Here's how the part is built. I have some questions about the finished solid (model axes, mm). A direction names the side the tool comes from. Coordinates: 2 decimals unless noted, no trailing zeros. Loops run counter-clockwise (first coordinate to the right, second up) from the corner with the lowest first, then second, coordinate; pieces in that order, holes last. Notation, with made-up numbers: M -11,66.25 L 9,66.25 A19 ccw 9,87.25 Z; hole C 77.5,66.5 d10. An arc over 180 degrees is marked long. Use CSV: the item, a comma, the result in double quotes. Start each with the question number.
Q1. Please list where these lines run through material, in increasing order: probe 1 along X at (y, z) = (3.5, 25); probe 2 along Z at (x, y) = (77.5, 6.25); probe 3 along X at (y, z) = (3.5, -15). Write a range as [from, to].
Q2. If we section it at A-A (x = 90): Please give me the cut outline in (y, z), and give its area (3 significant figures).
Q3. For pin 1 Ø2 at (x, z) = (100, 25) entering from +Y; pin 2 Ø4.5 at (x, z) = (-77.5, 14.5) entering from +Y, each with a flat end and sliding along its axis, tell me the tip position at first contact or that it passes through.
Q4. If we mould it in two halves opening along X, with no side actions, what happens to faces 6 (the flat face through (23, 10, -13)), 7 (the cylindrical face through (100.354, 3.402, -13.176))? For each: +X half, -X half, draft (parallel to the pull), parting line (faces both ways), or undercut.
Q5. Which directions (+Z, -Z, +X, -X, +Y, -Y) give clear straight access to the entire face, cutting with the end or side of a thin tool? Please do faces 1 (the flat face through (-2, 7, -2)), 2 (the cylindrical face through (92.1, 4.93, -15.09)), 3 (the cylindrical face through (73.004, 8.472, -12.698)), 4 (the flat face through (-2, 4, -40)), 5 (the flat face through (-2, 9, -29)).
Q6. If we section it at B-B (x = 5.5): Please give me the cut outline in (y, z).
Q7. If we section it at C-C (z = 30.5): Please give me the cut outline in (x, y).
from build123d import *

# Parameters (mm, degrees)
SKIZZE1_W                                            = 220
SKIZZE1_H                                            = 80
AUFSATZ_LINEAR_AUSTRAGEN1_DEPTH                      = 10
STIRNSENKUNG_F_R_M4_FLACHKOPFSCHRAUBE_MI_D           = 4.5
STIRNSENKUNG_F_R_M4_FLACHKOPFSCHRAUBE_MI_DEPTH       = 11.5
STIRNSENKUNG_F_R_M4_FLACHKOPFSCHRAUBE_MI_CBORE_D     = 9
STIRNSENKUNG_F_R_M4_FLACHKOPFSCHRAUBE_MI_CBORE_DEPTH = 3.1
STIRNSENKUNG_F_R_M4_FLACHKOPFSCHRAUBE_MI_TIP         = 1.351936393
M3_GEWINDEBOHRUNG1_AT_2_COUNT                        = 2
M3_GEWINDEBOHRUNG1_AT_2_PITCH                        = 50
M3_GEWINDEBOHRUNG1_AT_3_COUNT                        = 2
M3_GEWINDEBOHRUNG1_AT_3_PITCH                        = 100
M3_GEWINDEBOHRUNG1_AT_4_COUNT                        = 2
M3_GEWINDEBOHRUNG1_AT_4_PITCH                        = 150
M3_GEWINDEBOHRUNG1_AT_5_COUNT                        = 2
M3_GEWINDEBOHRUNG1_AT_5_PITCH                        = 50
M3_GEWINDEBOHRUNG1_AT_6_COUNT                        = 2
M3_GEWINDEBOHRUNG1_AT_6_PITCH                        = 200
M3_GEWINDEBOHRUNG1_AT_7_COUNT                        = 2
M3_GEWINDEBOHRUNG1_AT_7_PITCH                        = 250
SKIZZE8_W                                            = 15
SKIZZE8_H                                            = 3
SCHNITT_LINEAR_AUSTRAGEN1_DEPTH                      = 224.830292856
M5_GEWINDEBOHRUNG1_D                                 = 4.2
SKIZZE13_W                                           = 220
SKIZZE13_H                                           = 21
SCHNITT_LINEAR_AUSTRAGEN2_DEPTH                      = 1
M3_GEWINDEBOHRUNG2_D                                 = 2.5


with BuildPart() as part:
    # Skizze1 → Aufsatz-Linear austragen1 (new body)
    with BuildSketch(Plane(origin=(0, 0, 0), x_dir=(1, 0, 0), z_dir=(0, 1, 0))):
        Rectangle(SKIZZE1_W, SKIZZE1_H)
    extrude(amount=AUFSATZ_LINEAR_AUSTRAGEN1_DEPTH)

    # Stirnsenkung für M4 Flachkopfschraube mit Schlitz1
    with Locations(Plane(origin=(0, 10, 0), x_dir=(1, 0, 0), z_dir=(0, 1, 0))):
        with Locations((-102.5, 12.5), (-77.5, 12.5), (-77.5, -12.5), (-102.5, -12.5), (102.5, -12.5), (77.5, -12.5), (77.5, 12.5), (102.5, 12.5)):
            CounterBoreHole(STIRNSENKUNG_F_R_M4_FLACHKOPFSCHRAUBE_MI_D / 2, STIRNSENKUNG_F_R_M4_FLACHKOPFSCHRAUBE_MI_CBORE_D / 2, STIRNSENKUNG_F_R_M4_FLACHKOPFSCHRAUBE_MI_CBORE_DEPTH, depth=STIRNSENKUNG_F_R_M4_FLACHKOPFSCHRAUBE_MI_DEPTH)
            with Locations((0, 0, -(STIRNSENKUNG_F_R_M4_FLACHKOPFSCHRAUBE_MI_DEPTH + STIRNSENKUNG_F_R_M4_FLACHKOPFSCHRAUBE_MI_TIP / 2))):  # 118° drill point
                Cone(0, STIRNSENKUNG_F_R_M4_FLACHKOPFSCHRAUBE_MI_D / 2, STIRNSENKUNG_F_R_M4_FLACHKOPFSCHRAUBE_MI_TIP, mode=Mode.SUBTRACT)

    # Skizze7 → M3 Gewindebohrung1 (revolve, cut)
    with BuildSketch(Plane(origin=(-50, 10, -25), x_dir=(0, 0, 1), z_dir=(1, 0, 0))):
        Polygon((0, 0), (0, 9.251075774), (1.25, 8.5), (1.25, 0), align=None)
    m3_gewindebohrung1 = revolve(axis=Axis((-50, 16.35, -25), (0, -1, 0)), mode=Mode.SUBTRACT)

    # M3 Gewindebohrung1 at 2: M3 Gewindebohrung1 ×2
    with Locations(*[(i * M3_GEWINDEBOHRUNG1_AT_2_PITCH, 0, 0) for i in range(1, M3_GEWINDEBOHRUNG1_AT_2_COUNT)]):
        add(m3_gewindebohrung1, mode=Mode.SUBTRACT)

    # M3 Gewindebohrung1 at 3: M3 Gewindebohrung1 ×2
    with Locations(*[(i * M3_GEWINDEBOHRUNG1_AT_3_PITCH, 0, 0) for i in range(1, M3_GEWINDEBOHRUNG1_AT_3_COUNT)]):
        add(m3_gewindebohrung1, mode=Mode.SUBTRACT)

    # M3 Gewindebohrung1 at 4: M3 Gewindebohrung1 ×2
    with Locations(*[(i * M3_GEWINDEBOHRUNG1_AT_4_PITCH, 0, 0) for i in range(1, M3_GEWINDEBOHRUNG1_AT_4_COUNT)]):
        add(m3_gewindebohrung1, mode=Mode.SUBTRACT)

    # M3 Gewindebohrung1 at 5: M3 Gewindebohrung1 ×2
    with Locations(*[(-i * M3_GEWINDEBOHRUNG1_AT_5_PITCH, 0, 0) for i in range(1, M3_GEWINDEBOHRUNG1_AT_5_COUNT)]):
        add(m3_gewindebohrung1, mode=Mode.SUBTRACT)

    # M3 Gewindebohrung1 at 6: M3 Gewindebohrung1 ×2
    with Locations(*[(i * M3_GEWINDEBOHRUNG1_AT_6_PITCH, 0, 0) for i in range(1, M3_GEWINDEBOHRUNG1_AT_6_COUNT)]):
        add(m3_gewindebohrung1, mode=Mode.SUBTRACT)

    # M3 Gewindebohrung1 at 7: M3 Gewindebohrung1 ×2
    with Locations(*[(i * M3_GEWINDEBOHRUNG1_AT_7_PITCH, 0, 0) for i in range(1, M3_GEWINDEBOHRUNG1_AT_7_COUNT)]):
        add(m3_gewindebohrung1, mode=Mode.SUBTRACT)

    # Skizze8 → Schnitt-Linear austragen1 (cut, through all)
    with BuildSketch(Plane.ZY.offset(110)):
        with Locations((0, 8.5)):
            Rectangle(SKIZZE8_W, SKIZZE8_H)
    extrude(amount=-SCHNITT_LINEAR_AUSTRAGEN1_DEPTH, mode=Mode.SUBTRACT)

    # Spiegeln1: M3 Gewindebohrung1 across plane
    add(m3_gewindebohrung1.mirror(Plane.XY), mode=Mode.SUBTRACT)

    # Spiegeln1 copy 1 sketch → Spiegeln1 copy 1 (revolve, cut)
    with BuildSketch(Plane(origin=(0, 10, 25), x_dir=(0, 0, -1), z_dir=(1, 0, 0))):
        Polygon((0, 0), (0, -9.251075774), (1.25, -8.5), (1.25, 0), align=None)
    revolve(axis=Axis((0, 16.35, 25), (0, 1, 0)), mode=Mode.SUBTRACT)

    # Spiegeln1 copy 2 sketch → Spiegeln1 copy 2 (revolve, cut)
    with BuildSketch(Plane(origin=(50, 10, 25), x_dir=(0, 0, -1), z_dir=(1, 0, 0))):
        Polygon((0, 0), (0, -9.251075774), (1.25, -8.5), (1.25, 0), align=None)
    revolve(axis=Axis((50, 16.35, 25), (0, 1, 0)), mode=Mode.SUBTRACT)

    # Spiegeln1 copy 3 sketch → Spiegeln1 copy 3 (revolve, cut)
    with BuildSketch(Plane(origin=(100, 10, 25), x_dir=(0, 0, -1), z_dir=(1, 0, 0))):
        Polygon((0, 0), (0, -9.251075774), (1.25, -8.5), (1.25, 0), align=None)
    revolve(axis=Axis((100, 16.35, 25), (0, 1, 0)), mode=Mode.SUBTRACT)

    # Spiegeln1 copy 4 sketch → Spiegeln1 copy 4 (revolve, cut)
    with BuildSketch(Plane(origin=(-100, 10, 25), x_dir=(0, 0, -1), z_dir=(1, 0, 0))):
        Polygon((0, 0), (0, -9.251075774), (1.25, -8.5), (1.25, 0), align=None)
    revolve(axis=Axis((-100, 16.35, 25), (0, 1, 0)), mode=Mode.SUBTRACT)

    # Spiegeln1 copy 5 sketch → Spiegeln1 copy 5 (revolve, cut)
    with BuildSketch(Plane(origin=(150, 10, 25), x_dir=(0, 0, -1), z_dir=(1, 0, 0))):
        Polygon((0, 0), (0, -9.251075774), (1.25, -8.5), (1.25, 0), align=None)
    revolve(axis=Axis((150, 16.35, 25), (0, 1, 0)), mode=Mode.SUBTRACT)

    # Spiegeln1 copy 6 sketch → Spiegeln1 copy 6 (revolve, cut)
    with BuildSketch(Plane(origin=(200, 10, 25), x_dir=(0, 0, -1), z_dir=(1, 0, 0))):
        Polygon((0, 0), (0, -9.251075774), (1.25, -8.5), (1.25, 0), align=None)
    revolve(axis=Axis((200, 16.35, 25), (0, 1, 0)), mode=Mode.SUBTRACT)

    # M5 Gewindebohrung1 (through all)
    with Locations(Plane(origin=(0, 10, 0), x_dir=(1, 0, 0), z_dir=(0, 1, 0))):
        with Locations((90, -15), (90, 15), (-90, 15), (-90, -15), (0, 0)):
            Hole(M5_GEWINDEBOHRUNG1_D / 2)

    # Skizze13 → Schnitt-Linear austragen2 (cut)
    with BuildSketch(Plane(origin=(0, 10, 0), x_dir=(1, 0, 0), z_dir=(0, 1, 0))):
        with Locations((0, -29.5)):
            Rectangle(SKIZZE13_W, SKIZZE13_H)
    schnitt_linear_austragen2 = extrude(amount=-SCHNITT_LINEAR_AUSTRAGEN2_DEPTH, mode=Mode.SUBTRACT)

    # Spiegeln2: Schnitt-Linear austragen2 across plane
    add(schnitt_linear_austragen2.mirror(Plane.XY), mode=Mode.SUBTRACT)

    # M3 Gewindebohrung2 (through all)
    with Locations(Plane(origin=(-95, 7, 0), x_dir=(0, 0, 1), z_dir=(0, 1, 0))):
        with Locations((0, 0)):
            m3_gewindebohrung2 = Hole(M3_GEWINDEBOHRUNG2_D / 2)

    # Spiegeln3: M3 Gewindebohrung2 across plane
    add(m3_gewindebohrung2.mirror(Plane(origin=(0, 0, 0), x_dir=(0, 0, 1), z_dir=(1, 0, 0))), mode=Mode.SUBTRACT)


solid = part.part
Results below:
1,probe 1,"[-110, -101.25], [-98.75, -51.25], [-48.75, -1.25], [1.25, 48.75], [51.25, 98.75], [101.25, 110]"
1,probe 2,"[-40, -14.75], [-10.25, 10.25], [14.75, 40]"
1,probe 3,"[-110, -92.1], [-87.9, 87.9], [92.1, 110]"
2,outline,"M 0,-40 L 9,-40 L 9,-19 L 10,-19 L 10,-17.1 L 0,-17.1 Z; M 0,-12.9 L 10,-12.9 L 10,-7.5 L 7,-7.5 L 7,7.5 L 10,7.5 L 10,12.9 L 0,12.9 Z; M 0,17.1 L 10,17.1 L 10,19 L 9,19 L 9,40 L 0,40 Z"
2,area,"629 mm^2"
3,pin 1,"y = 1.35"
3,pin 2,"y = 6.9"
4,face 6,"draft"
4,face 7,"undercut"
5,face 1,"+X, -X, +Y"
5,face 2,"+Y, -Y"
5,face 3,"+Y"
5,face 4,"-Z, +X, -X, +Y, -Y"
5,face 5,"-Z, +X, -X, +Y"
6,outline,"M 0,-40 L 9,-40 L 9,-19 L 10,-19 L 10,-7.5 L 7,-7.5 L 7,7.5 L 10,7.5 L 10,19 L 9,19 L 9,40 L 0,40 Z"
7,outline,"M -110,0 L 110,0 L 110,9 L -110,9 Z"
